Geometry: final body of the model. Coordinates: model frame, mm. Give positions to 0.01 mm unless a question says otherwise; leave off trailing zeros. Order: outer loops, then holes, each group sorted by start corner. A loop starts at its lowest first (then second) coordinate and runs counter-clockwise, first axis right, second up. Notation, with made-up numbers: (-10.75, 42.25) - (13.25, 42.25) arc R24 ccw to (13.25, 64.25) - close; hole circle Ø11 at (15.5, -13). An arc over 180 degrees is marked (long way). Put each result on its own line as item: value. Start each with the question number.
1. Ray query, line 1 along Z through (x, y) = (64.5, 1.7); line 2 along X through (y, z) = (3.15, 10); line 3 along X through (y, z) = (2.3, 55.5). Return the intervals inside material, ascending. Write a range as from..to.
2. Section A-A on x = 121.5. Return the cut outline in (y, z), plus the area to 3 significant figures.
3. Section B-B on z = 43. Return the cut outline in (x, y).
4. Section C-C on y = 2.1. Return the cut outline in (x, z).
5. First-contact query: P1, Ø2, axis at y = 3, z = 25.5, coming from the -X side. Flat tip, straight axial feed; report the tip coordinate or a pass-through.
from build123d import *

# Parameters (mm, degrees)
SKETCH_1_W          = 360
SKETCH_1_H          = 70
EXTRUDE_1_DEPTH     = 4
CUT_EXTRUDE_1_DEPTH = 367.764229444
CUT_EXTRUDE_2_DEPTH = 367.764229444
SKETCH_4_W          = 310
SKETCH_4_H          = 35
SKETCH_4_W_2        = 2.5
CUT_EXTRUDE_3_DEPTH = 367.764229444


with BuildPart() as part:
    # 草图1 → 凸台-拉伸1 (new body)
    with BuildSketch(Plane(origin=(0, 0, 0), x_dir=(1, 0, 0), z_dir=(0, 1, 0))):
        with Locations((180, -35)):
            Rectangle(SKETCH_1_W, SKETCH_1_H)
    extrude(amount=EXTRUDE_1_DEPTH)

    # 草图2 → 切除-拉伸1 (cut, through all)
    with BuildSketch(Plane(origin=(0, 4, 0), x_dir=(1, 0, 0), z_dir=(0, 1, 0))):
        with BuildLine():
            Line((22.5, -55), (25, -55))
            Line((25, -55), (335, -55))
            Line((335, -55), (337.5, -55))
            ThreePointArc((337.5, -55), (336.767766953, -53.232233047), (335, -52.5))
            Line((335, -52.5), (25, -52.5))
            ThreePointArc((25, -52.5), (23.232233047, -53.232233047), (22.5, -55))
        make_face()
        with BuildLine():
            Line((335, -55), (25, -55))
            Line((25, -55), (22.5, -55))
            ThreePointArc((22.5, -55), (23.232233047, -56.767766953), (25, -57.5))
            Line((25, -57.5), (335, -57.5))
            ThreePointArc((335, -57.5), (336.767766953, -56.767766953), (337.5, -55))
            Line((337.5, -55), (335, -55))
        make_face()
    extrude(amount=-CUT_EXTRUDE_1_DEPTH, mode=Mode.SUBTRACT)

    # 草图3 → 切除-拉伸2 (cut, through all)
    with BuildSketch(Plane.XZ):
        with BuildLine():
            Line((25, 12.5), (335, 12.5))
            ThreePointArc((335, 12.5), (337.5, 10), (335, 7.5))
            Line((335, 7.5), (25, 7.5))
            ThreePointArc((25, 7.5), (22.5, 10), (25, 12.5))
        make_face()
    extrude(amount=-CUT_EXTRUDE_2_DEPTH, mode=Mode.SUBTRACT)

    # 草图4 → 切除-拉伸3 (cut, through all)
    with BuildSketch(Plane.XZ):
        with Locations((180, 32.5)):
            Rectangle(SKETCH_4_W, SKETCH_4_H)
        with Locations((23.75, 32.5)):
            Rectangle(SKETCH_4_W_2, SKETCH_4_H)
        with Locations((336.25, 32.5)):
            Rectangle(SKETCH_4_W_2, SKETCH_4_H)
    extrude(amount=-CUT_EXTRUDE_3_DEPTH, mode=Mode.SUBTRACT)


solid = part.part
Resolved:
1. line 1: 0..7.5, 12.5..15, 50..52.5, 57.5..70
1. line 2: 0..22.5, 337.5..360
1. line 3: 0..22.55, 337.45..360
2. outline: (0, 0) - (4, 0) - (4, 7.5) - (0, 7.5) - close; (0, 12.5) - (4, 12.5) - (4, 15) - (0, 15) - close; (0, 50) - (4, 50) - (4, 52.5) - (0, 52.5) - close; (0, 57.5) - (4, 57.5) - (4, 70) - (0, 70) - close
2. area: 100 mm^2
3. outline: (0, 0) - (22.5, 0) - (22.5, 4) - (0, 4) - close; (337.5, 0) - (360, 0) - (360, 4) - (337.5, 4) - close
4. outline: (0, 0) - (360, 0) - (360, 70) - (0, 70) - close; hole (22.5, 15) - (337.5, 15) - (337.5, 50) - (22.5, 50) - close; hole (25, 7.5) - (335, 7.5) arc R2.5 ccw to (335, 12.5) - (25, 12.5) arc R2.5 ccw to start; hole (25, 52.5) - (335, 52.5) arc R2.5 ccw to (335, 57.5) - (25, 57.5) arc R2.5 ccw to start
5. P1: x = 0
